Geometry check sheet. Reference: the model listing, model coordinates, mm. Coordinates: 2 decimals unless noted, no trailing zeros. Write each loop counter-clockwise with the first axis right and the second up, starting at its lowest first coordinate (ties: lowest second). Pieces come first, ordered by that corner, then holes. Notation, with made-up numbers: (-5.75, 10) - (29.25, 10) arc R6 cw to (29.25, 14) - close; hole circle Ø2 at (1, -2). An arc over 180 degrees is marked (long way). Answer as a JSON object with one key per item and string values. Group by question number.
from build123d import *

# Parameters (mm, degrees)
SKETCH046_W             = 550
SKETCH046_H             = 6
PAD009_DEPTH            = 32
SKETCH047_R             = 6
POCKET004_DEPTH         = 6.001
LINEARPATTERN002_COUNT  = 4
LINEARPATTERN002_PITCH  = 170
BODY006_PLACEMENT_ANGLE = 325


with BuildPart() as part:
    # Sketch046 → Pad009 (new body)
    with BuildSketch(Plane.XY):
        with Locations((275, 3)):
            Rectangle(SKETCH046_W, SKETCH046_H)
    extrude(amount=PAD009_DEPTH)

    # Sketch047 (on Face1 of Pad009) → Pocket004 (cut, through all)
    with BuildSketch(Plane.XZ):
        with Locations((20, 16)):
            Circle(SKETCH047_R)
    pocket004 = extrude(amount=-POCKET004_DEPTH, mode=Mode.SUBTRACT)

    # LinearPattern002: Pocket004 ×4
    with Locations(*[(i * LINEARPATTERN002_PITCH, 0, 0) for i in range(1, LINEARPATTERN002_COUNT)]):
        add(pocket004, mode=Mode.SUBTRACT)


with BuildPart() as part_1:
    # Body006 placement: moved
    add(part.part.moved(Location((-460.212515, 336.893567, 18))).rotate(Axis((-460.212515, 336.893567, 18), (0, 0, 1)), BODY006_PLACEMENT_ANGLE))


solid = part_1.part
(1) Material ranges on L1, parallel to Y at x = -393, z = 45; L2, parallel to Y at x = -327, z = 35; L3, parallel to X at y = 228, z = 42.5, recorded low to high. Write a range as [from, to].
(2) Gauge pin test, flat ends, axial feed: pin 1 (6 mm diameter, centred on y = 176.5, z = 21.5, fed in from -X); pin 2 (8 mm diameter, centred on x = -156.5, z = 42.5, fed in from +Y); pin 3 (6 mm diameter, centred on x = -158.5, z = 30.5, fed in from +Y). Record the tip position at first contact, or that the pin passes through.
(3) Section check A-A (y = 273.5). Record the cut outline in (x, z).
(4) Draft check along X on faces 1 (the face through (-234.658, 186.283, 33.776)), 2 (the face through (-167.52, 135.56, 30.35)), 3 (the face through (-238.1, 181.37, 33.78)). Enter one of: +X half, -X half, draft (parallel to the pull), parting line (faces both ways), or undercut.
(5) Section check B-B (x = -43.5). Record the cut outline in (y, z), and give its area (3 significant figures).
Conclusion:
{
 "1": {"L1": "y = [289.83, 297.16]", "L2": "y = [243.62, 250.94]", "L3": "x = [-304.7, -294.24]"},
 "2": {"pin 1": "stops at x = -235.43", "pin 2": "stops at y = 134.36", "pin 3": "stops at y = 134.34"},
 "3": {"outline": "(-369.68, 18) - (-359.22, 18) - (-359.22, 50) - (-369.68, 50) - close"},
 "4": {"face 1": "+X half", "face 2": "undercut", "face 3": "-X half"},
 "5": {"outline": "(45.11, 18) - (52.43, 18) - (52.43, 50) - (45.11, 50) - close", "area": "234 mm^2"}
}
